Can you work these out from the model? Positions are in its coordinate system, mm. A direction names the side the tool comes from. Round coordinates to 2 decimals unless told otherwise and drop trailing zeros. Loops run counter-clockwise (first coordinate to the right, second up) from the corner with the lowest first, then second, coordinate; pieces in that order, holes last. Notation, with made-up numbers: (50, 5) -> (90, 5) arc R8 ccw to (90, 9) -> close; hole circle Ø3 at (21.5, 76). An arc over 180 degrees is marked (long way). Answer as a JSON object with one key per item and string values.
```python
from build123d import *

# Parameters (mm, degrees)
BOSS_EXTRUDE1_DEPTH                                 = 65
BOSS_EXTRUDE2_START                                 = -15
SKETCH2_R                                           = 32.5
BOSS_EXTRUDE2_DEPTH                                 = 15
SKETCH3_R                                           = 20
BOSS_EXTRUDE4_DEPTH                                 = 25
CBORE_FOR_1_BINDING_HEAD_MACHINE_SCREW1_D           = 13.499999924
CBORE_FOR_1_BINDING_HEAD_MACHINE_SCREW1_CBORE_D     = 23.789999918
CBORE_FOR_1_BINDING_HEAD_MACHINE_SCREW1_CBORE_DEPTH = 7.499999986


with BuildPart() as part:
    # Sketch1 → Boss-Extrude1 (new body)
    with BuildSketch(Plane.XY):
        Polygon((0, 0), (0, 15), (68, 15), (68, -15), (53, -15), (53, 0), align=None)
    extrude(amount=BOSS_EXTRUDE1_DEPTH)

    # Sketch2 → Boss-Extrude2 (add)
    with BuildSketch(Plane(origin=(0, 15, 0), x_dir=(1, 0, 0), z_dir=(0, 1, 0)).offset(BOSS_EXTRUDE2_START)):
        with Locations((0, -32.5)):
            Circle(SKETCH2_R)
    extrude(amount=BOSS_EXTRUDE2_DEPTH)

    # Sketch3 → Boss-Extrude4 (add)
    with BuildSketch(Plane(origin=(0, 15, 0), x_dir=(1, 0, 0), z_dir=(0, 1, 0))):
        with Locations(Location((0, -32.5, 0), (0, 0, 90))):
            Circle(SKETCH3_R)
    extrude(amount=BOSS_EXTRUDE4_DEPTH)

    # CBORE for #1 Binding Head Machine Screw1 (through all)
    with Locations(Plane(origin=(0, 40, 0), x_dir=(1, 0, 0), z_dir=(0, 1, 0))):
        with Locations((0, -32.5)):
            CounterBoreHole(CBORE_FOR_1_BINDING_HEAD_MACHINE_SCREW1_D / 2, CBORE_FOR_1_BINDING_HEAD_MACHINE_SCREW1_CBORE_D / 2, CBORE_FOR_1_BINDING_HEAD_MACHINE_SCREW1_CBORE_DEPTH)


solid = part.part
```
Q1. If I drill on L1, parallel to X at y = 38, z = 32; L2, parallel to Z at x = 0, y = 14; L3, parallel to X at y = 18, z = 32, over which ranges is the centre line in solid material (lowest first)? Write a range as [from, to].
Determined:
{"L1": "[-19.99, -11.88], [11.88, 19.99]", "L2": "[0, 25.75], [39.25, 65]", "L3": "[-19.99, -6.73], [6.73, 19.99]"}
Q2. I want a section at A-A, the plane z = 32.5. Write out the boundary of the cut face in (x, y) (3 decimals), then the cut area to 3 significant figures.
Determined:
{"outline": "(-32.5, 0) -> (-6.75, 0) -> (-6.75, 32.5) -> (-11.895, 32.5) -> (-11.895, 40) -> (-20, 40) -> (-20, 15) -> (-32.5, 15) -> close; (6.75, 0) -> (53, 0) -> (53, -15) -> (68, -15) -> (68, 15) -> (20, 15) -> (20, 40) -> (11.895, 40) -> (11.895, 32.5) -> (6.75, 32.5) -> close", "area": "2,120 mm²"}
Q3. I'm going to push flat-ended pins straight in: pin 1 (19 mm diameter, centred on x = -3, z = 32, fed in from +Y); pin 2 (6 mm diameter, centred on x = 57.5, y = 20, fed in from +Z); pin 3 (7.5 mm diameter, centred on y = -4, z = 39, fed in from -X); pin 4 (15.5 mm diameter, centred on x = 0, z = 32.5, fed in from -Y). Where does each tip first touch, or does it pass through?
Determined:
{"pin 1": "y = 40", "pin 2": "through", "pin 3": "x = 53", "pin 4": "y = 0"}
Q4. On a 3-axis mill with a long thin cutter (end or side, diameter ignored), from which of +Z, -Z, +X, -X, +Y, -Y can I reach the whole of each face in a straight line? I mean faces 1 (the flat face through (42, 4, 65)), 2 (the flat face through (5, 32.5, 38)), 3 (the flat face through (11, 0, 32)). Say none if no direction works.
Determined:
{"face 1": "+Z, +X, -X, +Y, -Y", "face 2": "+Y", "face 3": "+Z, -Z, -X, -Y"}
Q5. I want a section at C-C, the plane x = -9. Write out the boundary of the cut face in (y, z).
Determined:
{"outline": "(0, 1.27) -> (15, 1.27) -> (15, 14.64) -> (40, 14.64) -> (40, 24.72) -> (32.5, 24.72) -> (32.5, 40.28) -> (40, 40.28) -> (40, 50.36) -> (15, 50.36) -> (15, 63.73) -> (0, 63.73) -> close"}
Q6. I want a section at B-B, the plane y = 19. Write out the boundary of the cut face in (x, z).
Determined:
{"outline": "circle Ø40 at (0, 32.5); hole circle Ø13.5 at (0, 32.5)"}
Q7. We'd pull the mould along Z, two halves only. Please class faces 4 (the cylindrical face through (-6.007, 27.325, 13.424)), 5 (the flat face through (42, 4, 0)), 6 (the cylindrical face through (0.879, 16.023, 25.807)): pulls with the +Z half, pulls with the -Z half, needs draft (parallel to the pull), parting line crosses it, or undercut.
Determined:
{"face 4": "parting line crosses it", "face 5": "pulls with the -Z half", "face 6": "undercut"}
Q8. I want a section at D-D, the plane z = 50. Write out the boundary of the cut face in (x, y), then the cut area to 3 significant figures.
Determined:
{"outline": "(-27.39, 0) -> (53, 0) -> (53, -15) -> (68, -15) -> (68, 15) -> (9.68, 15) -> (9.68, 40) -> (-9.68, 40) -> (-9.68, 15) -> (-27.39, 15) -> close", "area": "2,140 mm²"}
